Can you work these out from the drawing? Everything is in mm from the part's minimum corner. A direction names the side the tool comes from. Coordinates: 2 decimals unless noted, no trailing zeros. Order: outer loops, then holes, each group sorted by start corner. A loop starts at its lowest first (then second) coordinate and runs counter-clockwise, first axis right, second up. Notation, with made-up numbers: (-26, -15.75) - (9, -15.75) arc R11 cw to (9, -9.75) - close; hole circle Ø4 at (43, 28.25). An arc over 180 degrees is marked (long way). Use a Markdown table: item, result. Add a question column.
(1) I want a section at A-A (y = 10.25). List the corners of the cut face in (x, z) for me, and give its area (3 significant figures).
(2) For pin 1 Ø0.7 at (y, z) = (16.5, 1.5) entering from +X; pin 2 Ø0.5 at (y, z) = (17, 2) entering from -X; pin 3 Ø0.9 at (x, y) = (3, 16.5) entering from -Z, each with a flat end and sliding along its axis, tell me the tip position at first contact or that it passes through.
(3) If I drill on L1, parallel to Y at x = 0.7, z = 2.2; L2, parallel to Y at x = 2.3, z = 2.1; L3, parallel to X at y = 3.5, z = 2.1, over which ranges is the centre line in solid material (lowest first)? Write a range as [from, to].
(4) On a 3-axis mill with a long thin cutter (end or side, diameter ignored), from which of +Z, -Z, +X, -X, +Y, -Y can I reach the whole of each face in a straight line? I mean the marked faces 1 and 2. Say none if no direction works.
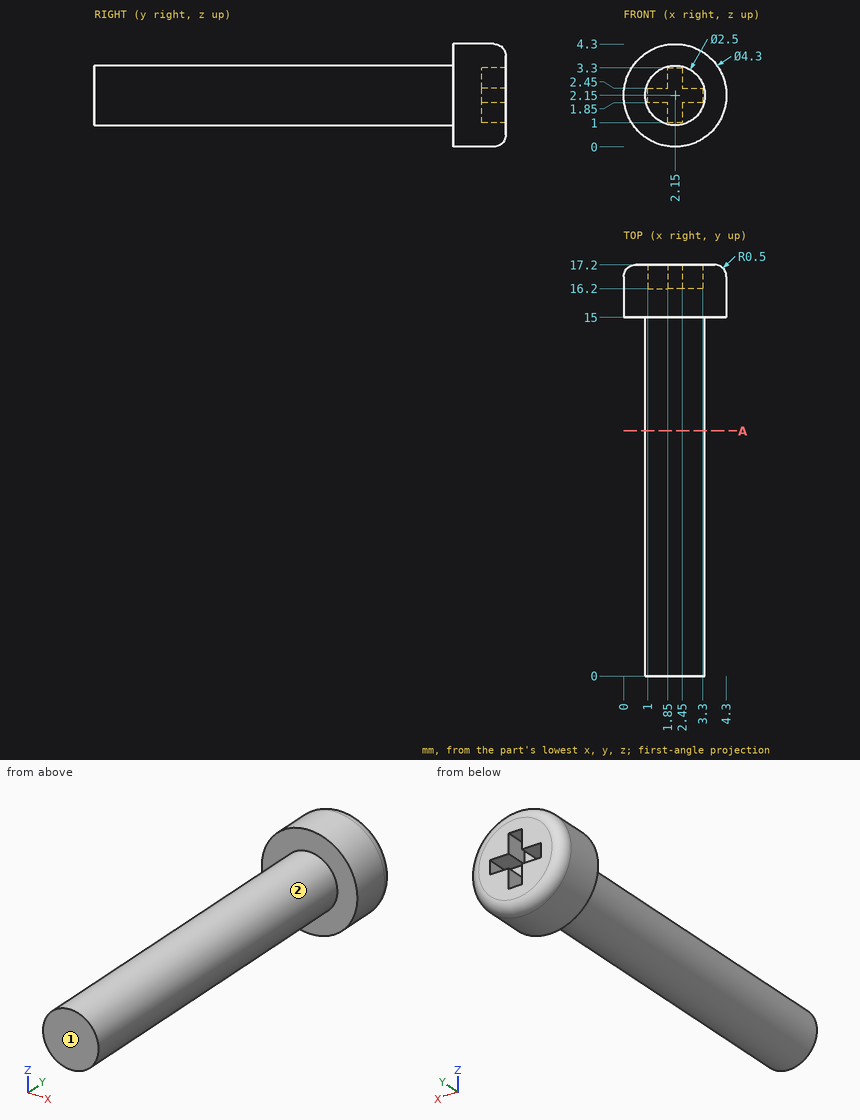
Answers follow:
| question | item | result |
|---|---|---|
| 1 | outline | circle Ø2.5 at (2.15, 2.15) |
| 1 | area | 4.91 mm² |
| 2 | pin 1 | stops at x = 4.28 |
| 2 | pin 2 | stops at x = 0.01 |
| 2 | pin 3 | stops at z = 0.04 |
| 3 | L1 | y = [15, 17.2] |
| 3 | L2 | y = [0, 16.2] |
| 3 | L3 | x = [0.9, 3.4] |
| 4 | face 1 | +Z, -Z, +X, -X, -Y |
| 4 | face 2 | -Y |
